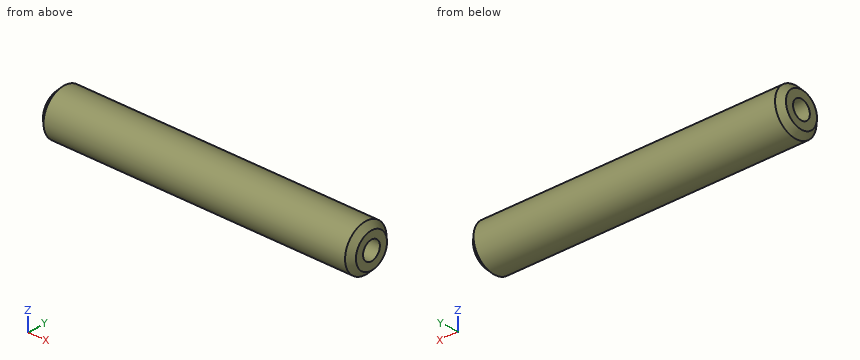
Solid Edge part; units mm, degrees
sketch "Sketch1" plane through (0, 0, 0) normal (0, -1, 0) x (1, 0, 0)
  line L0 (27.5, 0) -> (27.5, 4)
  line L1 (27.5, 4) -> (-27.5, 4)
  line L2 (-27.5, 4) -> (-27.5, 0)
  dimension "D1" = 27.5
revolve "RevolvedProtrusion1" add sketch "Sketch1" angle 360 about axis through (-32.5, 0, 0) along (1, 0, 0)
chamfer "Chamfer1" distance 1 angle 45 2 edges at (27.5, 0, -4) (-27.5, 0, -4)
hole "Hole_1" at (-27.5, 0, 0) direction (1, 0, 0) diameter 3.242 depth 20 tip angle 118 thread major 4 thread length 15
mirror "Mirror1" about plane through (0, 0, 0) normal (1, 0, 0) of "Hole_1"
properties material "AlSi7Mg"
Here's how the part is built. I have some questions about the finished solid (model axes, mm). Coordinates: 2 decimals unless noted, no trailing zeros. Write each loop counter-clockwise with the first axis right and the second up, starting at its lowest first coordinate (ties: lowest second). Pieces come first, ordered by that corner, then holes.
1) If I drill on line 1 (Y direction, x = -13.5, z = 0); line 2 (Y direction, x = 22, z = -1.25), over which ranges is the centre line in solid material (lowest first)?
Filled in:
line 1: y = -4 to -1.62, 1.62 to 4
line 2: y = -3.8 to -1.03, 1.03 to 3.8
2) If we section it at B-B (x = 2): List the corners of the cut face in (y, z) for me, plus the area to 3 significant figures.
Filled in:
outline: circle Ø8 at (0, 0)
area: 50.3 mm2
3) If we section it at A-A (x = 19.5): List the corners of the cut face in (y, z) for me, plus the area to 3 significant figures.
Filled in:
outline: circle Ø8 at (0, 0); hole circle Ø3.24 at (0, 0)
area: 42.0 mm2
4) I'm going to push flat-ended pins straight in: pin 1 (3 mm diameter, centred on x = 13.5, y = -2, fed in from -Z); pin 2 (1.5 mm diameter, centred on x = 0, z = -1, fed in from -Y). Where does each tip first touch, or does it pass through?
Filled in:
pin 1: stops at z = -3.97
pin 2: stops at y = -3.99
